Read the model definition and answer for the solid it produces. Units are mm, in the model's axes. A direction names the side the tool comes from. Round coordinates to 2 decimals unless told otherwise and drop trailing zeros. Write each loop counter-clockwise with the first axis right and the second up, starting at its lowest first coordinate (ties: lowest second). Pieces come first, ordered by that corner, then holes. Notation, with made-up numbers: (6.25, 35.5) - (31.25, 35.5) arc R21 cw to (31.25, 41.5) - close; hole circle Ø5 at (79.25, 77). An arc over 180 degrees is marked (long way). Use one line per item in the form item = value. Start each with the question number.
1) Each of these flat-tipped pins is pushed along its axis until it touches: pin 1 (6 mm diameter, centred on y = 28, z = -1, fed in from -X); pin 2 (5 mm diameter, centred on y = 44, z = 0, fed in from +X); pin 3 (6 mm diameter, centred on y = 40.5, z = -4, fed in from +X); pin 4 (4 mm diameter, centred on y = 24.5, z = -6.5, fed in from -X). Where does it stop, or does it pass through?
2) The part is cut by section C-C, the plane z = -1.5. Give the vertices of the cut face in (x, y), plus the area to 3 significant figures.
3) The part is cut by section A-A, the plane y = 27.5. Give the vertices of the cut face in (x, z), plus the area to 3 significant figures.
4) Consider line 1 along Y through (x, z) = (-131, 0.75); line 2 along Z through (x, y) = (-128.5, 18); line 3 along Y through (x, z) = (-119, -3.75). Determine where each line is inside the solid, lowest interval first. Write a range as from..to.
5) For a pull along X with two mould halves and no side action, classify faces 5 (the face through (-117.561, 36, 1)), 6 (the face through (-135.563, 18.636, 2.24)), 7 (the face through (-120, 19, -7.76)) as released by +X, released by -X, zero draft, split by the parting line, or undercut.
6) For faces 1 (the face through (-122.561, 36, 1)), 2 (the face through (-118.563, 48.636, 2.24)), 3 (the face through (-119.75, 28.92, -3.83)), 4 (the face through (-112, 21.071, 1)), determine the directions among +Z, -Z, +X, -X, +Y, -Y from which every point of the face is accessible in a straight line to the end or side of a thin tool.
7) The part is cut by section B-B, the plane x = -111.5. Give the vertices of the cut face in (y, z), plus the area to 3 significant figures.
8) The part is cut by section D-D, the plane y = 19. Give the vertices of the cut face in (x, z), plus the area to 3 significant figures.
from build123d import *

# Parameters (mm, degrees)
BOSS_EXTRUDE2_DEPTH = 1.5
SKETCH5_R           = 1.5
BOSS_EXTRUDE5_DEPTH = 3
SKETCH6_R           = 2.4
BOSS_EXTRUDE6_DEPTH = 7.76


with BuildPart() as part:
    # Sketch4 → Boss-Extrude2 (new body)
    with BuildSketch(Plane.XY):
        Polygon((-139.561248012, 16.070535031), (-106.561248012, 16.070535031), (-106.561248012, 21.070535031), (-117.561248012, 21.070535031), (-117.561248012, 51.070535031), (-122.561248012, 51.070535031), (-122.561248012, 21.070535031), (-139.561248012, 21.070535031), align=None)
    extrude(amount=BOSS_EXTRUDE2_DEPTH)

    # Sketch5 → Boss-Extrude5 (add)
    with BuildSketch(Plane(origin=(0, 0, 0), x_dir=(-1, 0, 0), z_dir=(0, 0, -1))):
        with Locations((137.061248012, 18.570535031)):
            Circle(SKETCH5_R)
        with Locations((109.061248012, 18.570535031)):
            Circle(SKETCH5_R)
        with Locations((120.061248012, 48.570535031)):
            Circle(SKETCH5_R)
    extrude(amount=-BOSS_EXTRUDE5_DEPTH)

    # Sketch6 → Boss-Extrude6 (add)
    with BuildSketch(Plane(origin=(0, 0, 0), x_dir=(-1, 0, 0), z_dir=(0, 0, -1))):
        with Locations((120.061248012, 18.570535031)):
            Circle(SKETCH6_R)
        with Locations((120.061248012, 26.540535031)):
            Circle(SKETCH6_R)
    extrude(amount=BOSS_EXTRUDE6_DEPTH)


solid = part.part
Geometry results:
q1.pin_1 = -122.56
q1.pin_2 = -117.56
q1.pin_3 = through
q1.pin_4 = -122.46
q2.outline = circle Ø4.8 at (-120.06, 18.57); circle Ø4.8 at (-120.06, 26.54)
q2.area = 36.2 mm2
q3.outline = (-122.56, 0) - (-122.26, 0) - (-122.26, -7.76) - (-117.86, -7.76) - (-117.86, 0) - (-117.56, 0) - (-117.56, 1.5) - (-122.56, 1.5) - close
q3.area = 41.6 mm2
q4.line_1 = 16.07..21.07
q4.line_2 = 0..1.5
q4.line_3 = 16.42..20.72, 24.39..28.69
q5.face_5 = released by +X
q5.face_6 = undercut
q5.face_7 = zero draft
q6.face_1 = +Z, -Z, -X, +Y
q6.face_2 = +Z
q6.face_3 = -Z
q6.face_4 = +Z, -Z, +X, +Y
q7.outline = (16.07, 0) - (21.07, 0) - (21.07, 1.5) - (16.07, 1.5) - close
q7.area = 7.50 mm2
q8.outline = (-139.56, 0) - (-122.42, 0) - (-122.42, -7.76) - (-117.7, -7.76) - (-117.7, 0) - (-106.56, 0) - (-106.56, 1.5) - (-107.62, 1.5) - (-107.62, 3) - (-110.5, 3) - (-110.5, 1.5) - (-135.62, 1.5) - (-135.62, 3) - (-138.5, 3) - (-138.5, 1.5) - (-139.56, 1.5) - close
q8.area = 94.8 mm2
